Input: part model. Units: mm. Frame: model coordinates. A direction names the side the tool comes from. Coordinates: 2 decimals unless noted, no trailing zeros. Write each loop counter-clockwise with the first axis right and the second up, starting at its lowest first coordinate (ties: lowest second). Pieces come first, ordered by that corner, then holes. Notation, with made-up numbers: (-33.5, -20.5) - (-1.5, -20.5) arc R31 ccw to (-1.5, 6.5) - close; hole circle Ø4 at (24.5, 12.25). An arc over 180 degrees is marked (long way). Put each result on its own line as item: value. Start each with the question number.
1. Line query: line 1 (Z direction, x = -71, y = -13); line 2 (Y direction, x = -92, z = 72.5); line 3 (X direction, y = -12, z = 110.5). Output: solid intervals per line, ascending.
2. Cut plane A-A, the plane y = -29.5. Return loops of the section in (x, z), and give its area (3 significant figures).
3. Cut plane B-B, the plane z = 60.5. Return loops of the section in (x, y).
4. Pin query (flat end, axial travel): pin 1 (16.5 mm diameter, centred on y = -36, z = 61.5, fed in from +X); pin 2 (1.5 mm diameter, centred on x = -74, y = -26, fed in from -Z). Return the tip coordinate at first contact, or that it passes through.
5. Access query for faces 1 (the flat face through (-111.342, -29, 101)), 2 (the flat face through (-103.959, -31, 97)). Directions: +Z, -Z, +X, -X, +Y, -Y. A direction counts if a zero-diameter tool reaches every point of the face in a straight line with its end or side. Return the directions, or none.
from build123d import *

# Parameters (mm, degrees)
SKETCH1_R           = 28.1
BOSS_EXTRUDE1_DEPTH = 1
SKETCH2_R           = 18.6
CUT_EXTRUDE1_DEPTH  = 58.8
SKETCH3_W           = 222.683092022
SKETCH3_H           = 364.2827524
BOSS_EXTRUDE2_DEPTH = 58.8
SKETCH4_W           = 207.917403516
SKETCH4_H           = 348.54429772
CUT_EXTRUDE2_DEPTH  = 55.8
SKETCH9_R           = 3
CUT_EXTRUDE8_DEPTH  = 10
SKETCH10_R          = 3.75
CUT_EXTRUDE9_DEPTH  = 10
CUT_EXTRUDE13_DEPTH = 500
SKETCH6_R           = 3.75
CUT_EXTRUDE5_DEPTH  = 400
SKETCH8_R           = 10
CUT_EXTRUDE7_DEPTH  = 10


with BuildPart() as part:
    # Sketch1 → Boss-Extrude1 (new body)
    with BuildSketch(Plane(origin=(0, 0, 0), x_dir=(1, 0, 0), z_dir=(0, 1, 0))):
        Circle(SKETCH1_R)
    extrude(amount=BOSS_EXTRUDE1_DEPTH)

    # Sketch2 → Cut-Extrude1 (cut)
    with BuildSketch(Plane(origin=(0, 1, 0), x_dir=(1, 0, 0), z_dir=(0, 1, 0))):
        with Locations((0, -7)):
            Circle(SKETCH2_R)
    extrude(amount=-CUT_EXTRUDE1_DEPTH, mode=Mode.SUBTRACT)

    # Sketch3 → Boss-Extrude2 (add)
    with BuildSketch(Plane(origin=(0, 0, 0), x_dir=(-1, 0, 0), z_dir=(0, -1, 0))):
        Rectangle(SKETCH3_W, SKETCH3_H)
    extrude(amount=BOSS_EXTRUDE2_DEPTH)

    # Sketch4 → Cut-Extrude2 (cut)
    with BuildSketch(Plane(origin=(0, -58.8, 0), x_dir=(-1, 0, 0), z_dir=(0, -1, 0))):
        Rectangle(SKETCH4_W, SKETCH4_H)
    extrude(amount=-CUT_EXTRUDE2_DEPTH, mode=Mode.SUBTRACT)

    # Sketch9 → Cut-Extrude8 (cut)
    with BuildSketch(Plane(origin=(0, 0, 0), x_dir=(1, 0, 0), z_dir=(0, 1, 0))):
        with Locations((0, -7)):
            Circle(SKETCH9_R)
    extrude(amount=-CUT_EXTRUDE8_DEPTH, mode=Mode.SUBTRACT)

    # Sketch10 → Cut-Extrude9 (cut)
    with BuildSketch(Plane(origin=(0, 1, 0), x_dir=(1, 0, 0), z_dir=(0, 1, 0))):
        with Locations((0, 19.85)):
            Circle(SKETCH10_R)
    extrude(amount=-CUT_EXTRUDE9_DEPTH, mode=Mode.SUBTRACT)

    # Sketch11 → Cut-Extrude13 (cut)
    with BuildSketch(Plane(origin=(0, -58.8, 0), x_dir=(-1, 0, 0), z_dir=(0, -1, 0))):
        Polygon((38.658453989, -17.8586238), (38.658453989, -182.1413762), (-111.341546011, -182.1413762), (-111.341546011, 182.1413762), (111.341546011, 182.1413762), (111.341546011, -17.8586238), align=None)
    extrude(amount=-CUT_EXTRUDE13_DEPTH, mode=Mode.SUBTRACT)

    # Sketch6 → Cut-Extrude5 (cut)
    with BuildSketch(Plane(origin=(0, 1, 0), x_dir=(1, 0, 0), z_dir=(0, 1, 0))):
        with Locations((0, 18.75)):
            Circle(SKETCH6_R)
    extrude(amount=-CUT_EXTRUDE5_DEPTH, mode=Mode.SUBTRACT)

    # Sketch8 → Cut-Extrude7 (cut)
    with BuildSketch(Plane(origin=(0, 0, -182.1413762), x_dir=(-1, 0, 0), z_dir=(0, 0, -1))):
        with Locations((-86.573671766, -25.011155335)):
            Circle(SKETCH8_R)
    extrude(amount=-CUT_EXTRUDE7_DEPTH, mode=Mode.SUBTRACT)


solid = part.part
Report:
1. line 1: z = 174.27 to 182.14
1. line 2: y = -3 to 0
1. line 3: x = -111.34 to -103.96
2. outline: (-111.34, 17.86) - (-103.96, 17.86) - (-103.96, 174.27) - (-38.66, 174.27) - (-38.66, 182.14) - (-111.34, 182.14) - close
2. area: 1,730 mm^2
3. outline: (-111.34, -58.8) - (-103.96, -58.8) - (-103.96, -3) - (-38.66, -3) - (-38.66, 0) - (-111.34, 0) - close
4. pin 1: stops at x = -103.96
4. pin 2: stops at z = 174.27
5. face 1: +Z, -Z, -X, +Y, -Y
5. face 2: -Z, +X, -Y
